```python
from build123d import *

# Parameters (mm, degrees)
SKETCH1_W   = 6.5
SKETCH1_H   = 3
SKETCH1_H_2 = 2
SKETCH1_H_3 = 7
SKETCH1_W_2 = 2


with BuildPart() as part:
    # Sketch1 → Revolve1 (revolve)
    with BuildSketch(Plane.XY):
        Polygon((2, 0), (2.5, 0), (2.5, 7), (2.5, 10), (2.5, 12), (2.5, 14), (2.5, 17), (2, 17), align=None)
        with Locations((5.75, 15.5)):
            Rectangle(SKETCH1_W, SKETCH1_H)
        with Locations((5.75, 11)):
            Rectangle(SKETCH1_W, SKETCH1_H_2)
        with Locations((5.75, 3.5)):
            Rectangle(SKETCH1_W, SKETCH1_H_3)
        with Locations((3.5, 8.5)):
            Rectangle(SKETCH1_W_2, SKETCH1_H)
        with Locations((3.5, 13)):
            Rectangle(SKETCH1_W_2, SKETCH1_H_2)
    revolve(axis=Axis((0, 0, 0), (0, 1, 0)))


solid = part.part
```
Check sheet for the modelled part. Datum: model origin and axes. Units: mm. A direction names the side the tool comes from. Give positions to 0.01 mm unless a question says otherwise; leave off trailing zeros. Loops run counter-clockwise (first coordinate to the right, second up) from the corner with the lowest first, then second, coordinate; pieces in that order, holes last. Notation, with made-up numbers: M 15,44.25 L 65,44.25 A21 ccw 65,65.25 Z; hole C -17,66.5 d3. An arc over 180 degrees is marked long. Answer in a Markdown table with one row per item.
1) Depth check by flat-ended pin: pin 1 (5 mm diameter, centred on y = 14.5, z = -5.5, fed in from +X); pin 2 (10 mm diameter, centred on y = 11, z = -4, fed in from -X); pin 3 (8 mm diameter, centred on y = 6.5, z = 5.5, fed in from -X); pin 4 (6 mm diameter, centred on y = 11, z = 5.5, fed in from +X). Enter the tip coordinate at first touch or a pass-through.
Solutions:
| item | result |
|---|---|
| pin 1 | stops at x = 8.49 |
| pin 2 | stops at x = -9 |
| pin 3 | stops at x = -8.87 |
| pin 4 | stops at x = 8.65 |
2) Cross-section at A-A (z = 0). Enter the section's corners in (x, y).
Solutions:
| item | result |
|---|---|
| outline | M -9,0 L -2,0 L -2,17 L -9,17 L -9,14 L -4.5,14 L -4.5,12 L -9,12 L -9,10 L -4.5,10 L -4.5,7 L -9,7 Z; M 2,0 L 9,0 L 9,7 L 4.5,7 L 4.5,10 L 9,10 L 9,12 L 4.5,12 L 4.5,14 L 9,14 L 9,17 L 2,17 Z |
3) Cross-section at D-D (z = -7.5). Enter the section's corners in (x, y), plus the area to 3 significant figures.
Solutions:
| item | result |
|---|---|
| outline | M -4.97,0 L 4.97,0 L 4.97,7 L -4.97,7 Z; M -4.97,10 L 4.97,10 L 4.97,12 L -4.97,12 Z; M -4.97,14 L 4.97,14 L 4.97,17 L -4.97,17 Z |
| area | 119 mm^2 |
4) Tool access check on faces 1 (the face through (-1.172, 15.521, -8.923)), 2 (the face through (-4, 12, 4)). Record the directions out of +Z, -Z, +X, -X, +Y, -Y that give a thin tool (end or side, any length) a straight path to the whole face; none if there is none.
Solutions:
| item | result |
|---|---|
| face 1 | +Y, -Y |
| face 2 | none |
5) Cross-section at C-C (x = 7.75). Enter the section's corners in (y, z).
Solutions:
| item | result |
|---|---|
| outline | M 0,-4.58 L 7,-4.58 L 7,4.58 L 0,4.58 Z; M 10,-4.58 L 12,-4.58 L 12,4.58 L 10,4.58 Z; M 14,-4.58 L 17,-4.58 L 17,4.58 L 14,4.58 Z |
6) Mould release check, pull along Z, two halves, no side actions. Record for faces 3 (the face through (-1.172, 11.014, -8.923)), 4 (the face through (-2, 0, 2)), 5 (the face through (0, 8, 2)): released by +Z, released by -Z, zero draft, split by the parting line, or undercut.
Solutions:
| item | result |
|---|---|
| face 3 | split by the parting line |
| face 4 | zero draft |
| face 5 | undercut |
7) Thickness scan on line 1 (Y direction, x = 4.5, z = 4.75); line 2 (X direction, y = 13, z = 0); line 3 (Z direction, x = 0, y = 11.25). Record the ranges inside material, lowest first.
Solutions:
| item | result |
|---|---|
| line 1 | y = 0 to 7, 10 to 12, 14 to 17 |
| line 2 | x = -4.5 to -2, 2 to 4.5 |
| line 3 | z = -9 to -2, 2 to 9 |
8) Cross-section at B-B (x = 0). Enter the section's corners in (y, z), plus the area to 3 significant figures.
Solutions:
| item | result |
|---|---|
| outline | M 0,-9 L 7,-9 L 7,-4.5 L 10,-4.5 L 10,-9 L 12,-9 L 12,-4.5 L 14,-4.5 L 14,-9 L 17,-9 L 17,-2 L 0,-2 Z; M 0,2 L 17,2 L 17,9 L 14,9 L 14,4.5 L 12,4.5 L 12,9 L 10,9 L 10,4.5 L 7,4.5 L 7,9 L 0,9 Z |
| area | 193 mm^2 |
